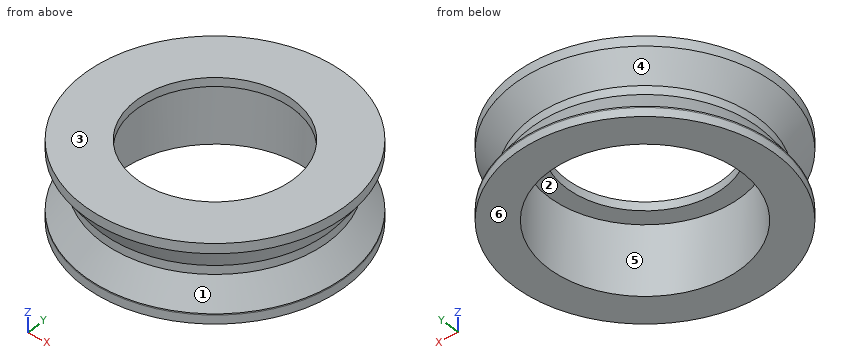
```python
from build123d import *

# Parameters (mm, degrees)
SKETCH2_R               = 13.02
SKETCH2_R_2             = 11.02
BOSS_EXTRUDE1_DEPTH     = 7
SKETCH3_R               = 15.02
SKETCH3_R_2             = 13.02
SKETCH3_R_3             = 11.02
SKETCH3_R_4             = 9
BOSS_EXTRUDE2_DEPTH     = 1
SALIENTE_EXTRUIR1_START = -8
SKETCH3_2_R             = 15.02
SKETCH3_2_R_2           = 13.02
SKETCH3_2_R_3           = 11.02
SALIENTE_EXTRUIR1_DEPTH = 1
CHAFL_N1_SIZE           = 3
CHAFL_N1_SIZE_2         = 2.100622615
CHAMFER1_SIZE           = 3
CHAMFER1_SIZE_2         = 2.100622615


with BuildPart() as part:
    # Sketch2 → Boss-Extrude1 (new body)
    with BuildSketch(Plane.XY):
        Circle(SKETCH2_R)
        Circle(SKETCH2_R_2, mode=Mode.SUBTRACT)
    extrude(amount=BOSS_EXTRUDE1_DEPTH)

    # Sketch3 → Boss-Extrude2 (add)
    # profile 1 of 3: a face of its own
    with BuildSketch(Plane.XY.offset(7)):
        Circle(SKETCH3_R)
        Circle(SKETCH3_R_2, mode=Mode.SUBTRACT)
    # profile 2 of 3: a face of its own
    with BuildSketch(Plane.XY.offset(7)):
        Circle(SKETCH3_R_2)
        Circle(SKETCH3_R_3, mode=Mode.SUBTRACT)
    # profile 3 of 3: a face of its own
    with BuildSketch(Plane.XY.offset(7)):
        Circle(SKETCH3_R_3)
        Circle(SKETCH3_R_4, mode=Mode.SUBTRACT)
    extrude(amount=BOSS_EXTRUDE2_DEPTH)

    # Sketch3<2> → Saliente-Extruir1 (add)
    # profile 1 of 2: a face of its own
    with BuildSketch(Plane.XY.offset(7).offset(SALIENTE_EXTRUIR1_START)):
        Circle(SKETCH3_2_R)
        Circle(SKETCH3_2_R_2, mode=Mode.SUBTRACT)
    # profile 2 of 2: a face of its own
    with BuildSketch(Plane.XY.offset(7).offset(SALIENTE_EXTRUIR1_START)):
        Circle(SKETCH3_2_R_2)
        Circle(SKETCH3_2_R_3, mode=Mode.SUBTRACT)
    extrude(amount=SALIENTE_EXTRUIR1_DEPTH)

    # Chaflán1
    # the kernel refuses this chamfer: 3, 2.100622615 mm, written as the material it adds along each edge
    with BuildSketch(Plane(origin=(0, 0, 7), x_dir=(1, 0, 0), z_dir=(0, -1, 0))) as chafl_n1_piece_1_section:
        Polygon((13.02, -CHAFL_N1_SIZE), (13.02 + CHAFL_N1_SIZE_2, 0), (13.02, 0), align=None)
    chafl_n1_piece_1 = revolve(axis=Axis((0, 0, 7), (0, 0, 1)), mode=Mode.PRIVATE)
    chafl_n1_piece_1 = chafl_n1_piece_1 & Plane(origin=(0, 0, 5.417457175), x_dir=(1, 0, 0), z_dir=(0, 0, -1)) * Cylinder(15.02, 61, mode=Mode.PRIVATE)
    add(chafl_n1_piece_1)

    # Chamfer1
    # the kernel refuses this chamfer: 3, 2.100622615 mm, written as the material it adds along each edge
    with BuildSketch(Plane(origin=(0, 0, 0), x_dir=(1, 0, 0), z_dir=(0, -1, 0))) as chamfer1_piece_1_section:
        Polygon((13.02, CHAMFER1_SIZE), (13.02 + CHAMFER1_SIZE_2, 0), (13.02, 0), align=None)
    chamfer1_piece_1 = revolve(axis=Axis((0, 0, 0), (0, 0, 1)), mode=Mode.PRIVATE)
    chamfer1_piece_1 = chamfer1_piece_1 & Plane(origin=(0, 0, 1.582542825), x_dir=(1, 0, 0), z_dir=(0, 0, -1)) * Cylinder(15.02, 61, mode=Mode.PRIVATE)
    add(chamfer1_piece_1)


solid = part.part
```
Can you work these out from the model? Positions are in its coordinate system, mm. Face numbers are marked on the shaded views. A direction names the side the tool comes from. Give positions to 0.01 mm unless a question says otherwise; leave off trailing zeros. Loops run counter-clockwise (first coordinate to the right, second up) from the corner with the lowest first, then second, coordinate; pieces in that order, holes last. Notation, with made-up numbers: M -7.5,15.25 L 2.5,15.25 A9 ccw 2.5,30.25 Z; hole C 20.5,-31 d8. An arc over 180 degrees is marked long. One line per question, with ' | ' between items. Start each with the question number.
Q1. For pin 1 Ø1.5 at (y, z) = (10, 4) entering from -X; pin 2 Ø1.5 at (x, z) = (-4, 6) entering from -Y; pin 3 Ø1 at (x, z) = (-6.5, 6) entering from -Y; pin 4 Ø5 at (x, z) = (-0.5, 1.5) entering from -Y, each with a flat end and sliding along its axis, tell me the tip position at first contact or that it passes through.
Q2. If we section it at A-A (y = 0): Please give me the cut outline in (x, z), plus the area to 3 significant figures.
Q3. If I drill on line 1 (Y direction, x = 0, z = 7.2); line 2 (Y direction, x = 0, z = 3.25); line 3 (Z direction, x = 8, y = 7), over which ranges is the centre line in solid material (lowest first)? Write a range as from..to.
Q4. For the marked faces 1, 2 and 3, which set-ups out of +Z, -Z, +X, -X, +Y, -Y let a thin tool reach every point of the face, with its end or its side?
Q5. If we mould it in two halves opening along Y, with no side actions, what happens to the marked faces 4, 5 and 6? For each: +Y half, -Y half, draft (parallel to the pull), parting line (faces both ways), or undercut.
Q6. If we section it at D-D (z = 6.25): Please give me the cut outline in (x, y).
Q7. If we section it at C-C (z = 3.5): Please give me the cut outline in (x, y).
Computed:
1) pin 1: stops at x = -9.47 | pin 2: stops at y = -14.44 | pin 3: stops at y = -13.33 | pin 4: stops at y = -15.02
2) outline: M -15.02,-1 L -11.02,-1 L -11.02,7 L -9,7 L -9,8 L -15.02,8 L -15.02,6.86 L -13.02,4 L -13.02,3 L -15.02,0.14 Z; M 9,7 L 11.02,7 L 11.02,-1 L 15.02,-1 L 15.02,0.14 L 13.02,3 L 13.02,4 L 15.02,6.86 L 15.02,8 L 9,8 Z | area: 60.6 mm²
3) line 1: y = -15.02..-9, 9..15.02 | line 2: y = -13.02..-11.02, 11.02..13.02 | line 3: z = 7..8
4) face 1: none | face 2: -Z | face 3: +Z, +X, -X, +Y, -Y
5) face 4: parting line | face 5: undercut | face 6: draft
6) outline: C 0,0 d29.19; hole C 0,0 d22.04
7) outline: C 0,0 d26.04; hole C 0,0 d22.04
